Drawing for the job (mm, zero at the part's lowest x, y, z). A direction names the side the tool comes from. Round coordinates to 2 decimals unless told otherwise and drop trailing zeros. Write each loop counter-clockwise with the first axis right and the second up, starting at its lowest first coordinate (ties: lowest second). Pieces come first, ordered by that corner, then holes. Notation, with made-up numbers: (42, 53.25) -> (78, 53.25) arc R24 cw to (78, 86.25) -> close; hole circle Ø2 at (39.25, 63). An arc over 180 degrees is marked (long way). One line per question, with ' | ' between items.
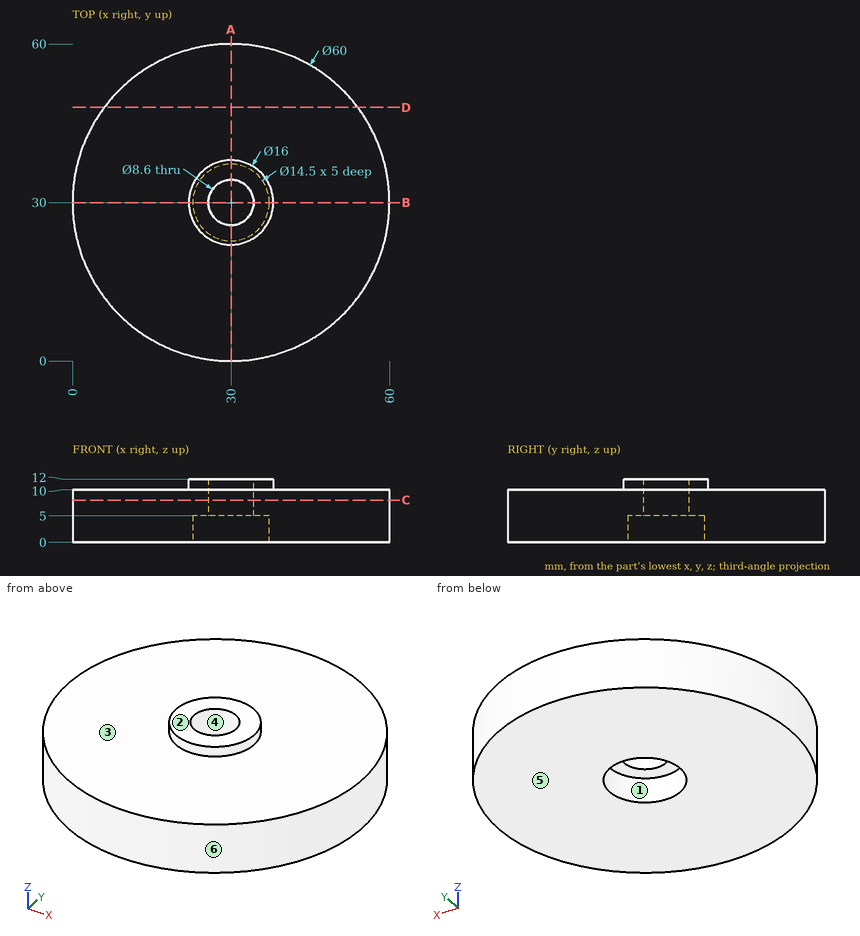
(1) Drop flat-ended pins along their axis: pin 1 (3 mm diameter, centred on y = 48, z = 5.5, fed in from -X); pin 2 (10 mm diameter, centred on x = 30, y = 30, fed in from +Z); pin 3 (5 mm diameter, centred on x = 43.5, z = 3, fed in from -Y); pin 4 (5 mm diameter, centred on y = 12, z = 6.5, fed in from +X). Give the stop position or say it passes through.
Calculated:
pin 1: x = 4.95 | pin 2: z = 12 | pin 3: y = 2.09 | pin 4: x = 55.69
(2) Slice it at A-A (x = 30). Write the cut outline in (y, z).
Calculated:
outline: (0, 0) -> (22.75, 0) -> (22.75, 5) -> (25.7, 5) -> (25.7, 12) -> (22, 12) -> (22, 10) -> (0, 10) -> close; (34.3, 5) -> (37.25, 5) -> (37.25, 0) -> (60, 0) -> (60, 10) -> (38, 10) -> (38, 12) -> (34.3, 12) -> close
(3) Slice it at D-D (y = 48). Write the cut outline in (x, z), then the cut area to 3 significant figures.
Calculated:
outline: (6, 0) -> (54, 0) -> (54, 10) -> (6, 10) -> close | area: 480 mm2
(4) Slice it at C-C (z = 8). Write the cut outline in (x, y).
Calculated:
outline: circle Ø60 at (30, 30); hole circle Ø8.6 at (30, 30)
(5) Wall check: line 1 (Y direction, x = 30, z = 3.35); line 2 (Y direction, x = 30, z = 9.5); line 3 (Z direction, x = 27, y = 39). Give the ranges that are in metal, low to high. Write a range as from..to.
Calculated:
line 1: 0..22.75, 37.25..60 | line 2: 0..25.7, 34.3..60 | line 3: 0..10
(6) Mould opens along Y. For the marked faces 4, 5 and 6 say: pulls with the +Y half, pulls with the -Y half, needs draft (parallel to the pull), parting line crosses it, or undercut.
Calculated:
face 4: undercut | face 5: needs draft | face 6: parting line crosses it
(7) 3-axis set-ups, long thin cutter, end or side, ignore diameter. For the marked faces 1, 2 and 3: which of +Z, -Z, +X, -X, +Y, -Y reach the whole face in a straight line?
Calculated:
face 1: -Z | face 2: +Z, +X, -X, +Y, -Y | face 3: +Z
